```python
from build123d import *

# Parameters (mm, degrees)
SKETCH_1_R          = 3.9
EXTRUDE_1_DEPTH     = 3
CHAMFER_1_SIZE      = 0.5
SKETCH_4_R          = 5.4
EXTRUDE_2_DEPTH     = 1
SKETCH_5_R          = 1.8
CUT_EXTRUDE_2_DEPTH = 2


with BuildPart() as part:
    # Эскиз1 → Бобышка-Вытянуть1 (new body)
    with BuildSketch(Plane.XY):
        Circle(SKETCH_1_R)
    extrude(amount=EXTRUDE_1_DEPTH)

    # Фаска1
    chamfer_1_edges = [part.edges().sort_by_distance(p)[0] for p in [
        (-3.9, 0, 0),
    ]]
    chamfer(chamfer_1_edges, length=CHAMFER_1_SIZE)

    # Эскиз4 → Бобышка-Вытянуть2 (add)
    with BuildSketch(Plane.XY.offset(3)):
        Circle(SKETCH_4_R)
    extrude(amount=EXTRUDE_2_DEPTH)

    # Эскиз5 → Вырез-Вытянуть2 (cut)
    with BuildSketch(Plane.XY.offset(4)):
        Circle(SKETCH_5_R)
    extrude(amount=-CUT_EXTRUDE_2_DEPTH, mode=Mode.SUBTRACT)


solid = part.part
```
Verification items for the finished model (mm, model axes). A direction names the side the tool comes from. Coordinates: 2 decimals unless noted, no trailing zeros. Loops run counter-clockwise (first coordinate to the right, second up) from the corner with the lowest first, then second, coordinate; pieces in that order, holes last. Notation, with made-up numbers: (81.5, 71) -> (93.5, 71) arc R23 ccw to (93.5, 95) -> close; hole circle Ø8 at (-20, -33.5). An arc over 180 degrees is marked (long way). Answer in a Markdown table with one row per item.
1) Section check C-C (z = 3.45). Record the cut outline in (x, y), and give its area (3 significant figures).
The answers:
| item | result |
|---|---|
| outline | circle Ø10.8 at (0, 0); hole circle Ø3.6 at (0, 0) |
| area | 81.4 mm2 |
2) Draft check along X on faces 1 (the face through (2, 0, 4)), 2 (the face through (-1.17, -5.27, 3.49)), 3 (the face through (0, 0, 2)). Enter one of: released by +X, released by -X, zero draft, split by the parting line, or undercut.
The answers:
| item | result |
|---|---|
| face 1 | zero draft |
| face 2 | split by the parting line |
| face 3 | undercut |
3) Section check A-A (y = 0). Record the cut outline in (x, z), and give its area (4 significant figures).
The answers:
| item | result |
|---|---|
| outline | (-5.4, 3) -> (-3.9, 3) -> (-3.9, 0.5) -> (-3.4, 0) -> (3.4, 0) -> (3.9, 0.5) -> (3.9, 3) -> (5.4, 3) -> (5.4, 4) -> (1.8, 4) -> (1.8, 2) -> (-1.8, 2) -> (-1.8, 4) -> (-5.4, 4) -> close |
| area | 26.75 mm2 |
4) Access from +Z, -Z, +X, -X, +Y, -Y to the whole of each face (thin tool, end or side, straight path). Record for faces 4 (the face through (1.717, 0.541, 3.014)), 5 (the face through (0, 0, 0)), 6 (the face through (-2.87, 2.64, 1.73)).
The answers:
| item | result |
|---|---|
| face 4 | +Z |
| face 5 | -Z, +X, -X, +Y, -Y |
| face 6 | -Z |
5) Section check D-D (z = 1.1). Record the cut outline in (x, y).
The answers:
| item | result |
|---|---|
| outline | circle Ø7.8 at (0, 0) |
6) Scan lines: line 1 along Y through (x, z) = (0, 3.15); line 2 along Y through (x, z) = (0, 2.95); line 3 along Z through (x, y) = (-0.75, 1.5). Record each from-to range of solid material in increasing order. Write a range as from..to.
The answers:
| item | result |
|---|---|
| line 1 | y = -5.4..-1.8, 1.8..5.4 |
| line 2 | y = -3.9..-1.8, 1.8..3.9 |
| line 3 | z = 0..2 |
7) Depth check by flat-ended pin: P1, Ø1.1, axis at x = 0, y = -0.5, coming from the +Z side; P2, Ø2, axis at y = 0, z = 1.5, coming from the +X side; P3, Ø1.5, axis at y = -3, z = 0.5, coming from the +X side. Enter the tip coordinate at first touch or a pass-through.
The answers:
| item | result |
|---|---|
| P1 | stops at z = 2 |
| P2 | stops at x = 3.9 |
| P3 | stops at x = 3.19 |
